Design review of the part built by this model. Coordinates are the model's own, in mm. Face numbers are marked on the shaded views. A direction names the side the tool comes from. Give positions to 0.01 mm unless a question says otherwise; leave off trailing zeros. Order: outer loops, then holes, each group sorted by start corner. A loop starts at its lowest first (then second) coordinate and runs counter-clockwise, first axis right, second up. Notation, with made-up numbers: (61.5, 36.5) -> (104.5, 36.5) arc R11 cw to (104.5, 53.5) -> close; hole circle Ø8 at (18, 71.5). An arc over 180 degrees is marked (long way). One line per item, written item: value.
from build123d import *

# Parameters (mm, degrees)
EXTRUDE_1_DEPTH     = 90
CUT_EXTRUDE_START   = -65
CUT_EXTRUDE_2_DEPTH = 65
SKETCH_4_R          = 2.1
CUT_EXTRUDE_3_DEPTH = 10


with BuildPart() as part:
    # Эскиз1 → Вытянуть1 (new body)
    with BuildSketch(Plane.XY):
        with BuildLine():
            Line((-17.5, 6.5), (-14.5, 6.5))
            ThreePointArc((-14.5, 6.5), (-13.792893219, 6.207106781), (-13.5, 5.5))
            Line((-13.5, 5.5), (-13.5, 2))
            ThreePointArc((-13.5, 2), (-12.914213562, 0.585786438), (-11.5, 0))
            Line((-11.5, 0), (11.5, 0))
            ThreePointArc((11.5, 0), (12.914213562, 0.585786438), (13.5, 2))
            Line((13.5, 2), (13.5, 5.5))
            ThreePointArc((13.5, 5.5), (13.792893219, 6.207106781), (14.5, 6.5))
            Line((14.5, 6.5), (17.5, 6.5))
            Line((17.5, 6.5), (17.5, 7.5))
            Line((17.5, 7.5), (14.5, 7.5))
            ThreePointArc((14.5, 7.5), (13.085786438, 6.914213562), (12.5, 5.5))
            Line((12.5, 5.5), (12.5, 2))
            ThreePointArc((12.5, 2), (12.207106781, 1.292893219), (11.5, 1))
            Line((11.5, 1), (-11.5, 1))
            ThreePointArc((-11.5, 1), (-12.207106781, 1.292893219), (-12.5, 2))
            Line((-12.5, 2), (-12.5, 5.5))
            ThreePointArc((-12.5, 5.5), (-13.085786438, 6.914213562), (-14.5, 7.5))
            Line((-14.5, 7.5), (-17.5, 7.5))
            Line((-17.5, 7.5), (-17.5, 6.5))
        make_face()
    extrude(amount=EXTRUDE_1_DEPTH)

    # Эскиз3 → Вырез-Вытянуть2 (cut)
    with BuildSketch(Plane.XY.offset(90).offset(CUT_EXTRUDE_START)):
        with BuildLine():
            Line((-17.5, 7.5), (-17.5, 6.5))
            Line((-17.5, 6.5), (-14.5, 6.5))
            ThreePointArc((-14.5, 6.5), (-13.792893219, 6.207106781), (-13.5, 5.5))
            Line((-13.5, 5.5), (-13.5, 2))
            ThreePointArc((-13.5, 2), (-12.914213562, 0.585786438), (-11.5, 0))
            Line((-11.5, 0), (11.5, 0))
            ThreePointArc((11.5, 0), (12.914213562, 0.585786438), (13.5, 2))
            Line((13.5, 2), (13.5, 5.5))
            ThreePointArc((13.5, 5.5), (13.792893219, 6.207106781), (14.5, 6.5))
            Line((14.5, 6.5), (17.5, 6.5))
            Line((17.5, 6.5), (17.5, 7.5))
            Line((17.5, 7.5), (14.5, 7.5))
            ThreePointArc((14.5, 7.5), (13.085786438, 6.914213562), (12.5, 5.5))
            Line((12.5, 5.5), (12.5, 2))
            ThreePointArc((12.5, 2), (12.207106781, 1.292893219), (11.5, 1))
            Line((11.5, 1), (-11.5, 1))
            ThreePointArc((-11.5, 1), (-12.207106781, 1.292893219), (-12.5, 2))
            Line((-12.5, 2), (-12.5, 5.5))
            ThreePointArc((-12.5, 5.5), (-13.085786438, 6.914213562), (-14.5, 7.5))
            Line((-14.5, 7.5), (-17.5, 7.5))
        make_face()
    extrude(amount=CUT_EXTRUDE_2_DEPTH, mode=Mode.SUBTRACT)

    # Эскиз4 → Вырез-Вытянуть3 (cut)
    with BuildSketch(Plane(origin=(0, 1, 0), x_dir=(-1, 0, 0), z_dir=(0, 1, 0))):
        with Locations((7.5, 7.5)):
            Circle(SKETCH_4_R)
        with Locations((-7.5, 17.5)):
            Circle(SKETCH_4_R)
    extrude(amount=-CUT_EXTRUDE_3_DEPTH, mode=Mode.SUBTRACT)


solid = part.part
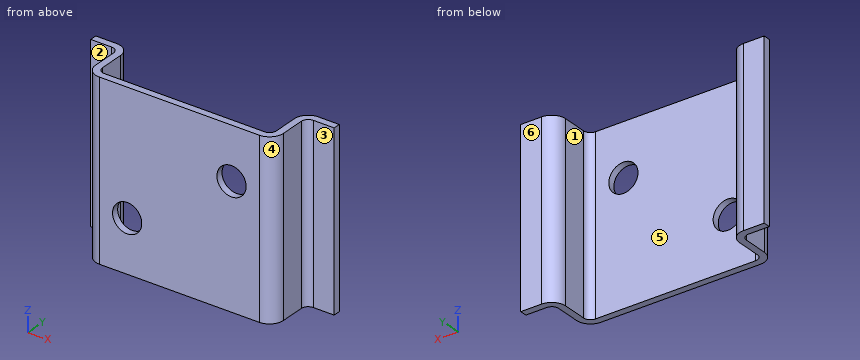
Item 1: Add section D-D on z = 4. Give the boundary of the cut face in (x, y).
Returned:
outline: (-17.5, 6.5) -> (-14.5, 6.5) arc R1 cw to (-13.5, 5.5) -> (-13.5, 2) arc R2 ccw to (-11.5, 0) -> (11.5, 0) arc R2 ccw to (13.5, 2) -> (13.5, 5.5) arc R1 cw to (14.5, 6.5) -> (17.5, 6.5) -> (17.5, 7.5) -> (14.5, 7.5) arc R2 ccw to (12.5, 5.5) -> (12.5, 2) arc R1 cw to (11.5, 1) -> (-11.5, 1) arc R1 cw to (-12.5, 2) -> (-12.5, 5.5) arc R2 ccw to (-14.5, 7.5) -> (-17.5, 7.5) -> close
Item 2: Draft analysis for pull direction X (two halves, no side actions). For the marked faces 4, 5 and 6, state which applies: pulls with the +X half, pulls with the -X half, needs draft (parallel to the pull), parting line crosses it, or undercut.
Returned:
face 4: pulls with the +X half
face 5: undercut
face 6: needs draft
Item 3: Add section C-C on x = -7.5. Give the boundary of the cut face in (y, z), plus the area to 3 significant figures.
Returned:
outline: (0, 0) -> (1, 0) -> (1, 5.4) -> (0, 5.4) -> close; (0, 9.6) -> (1, 9.6) -> (1, 25) -> (0, 25) -> close
area: 20.8 mm²
Item 4: Clearance check with flat-ended pins moving along their axes: P1, Ø3, axis at y = 4.5, z = 7, coming from the -X side; P2, Ø1, axis at x = -4, z = 16, coming from the +Y side; P3, Ø3.5, axis at x = -16.5, z = 14, coming from the -Y side. State where each tip first meets the part, or that it passes through.
Returned:
P1: x = -13.63
P2: y = 1
P3: y = 6.5
Item 5: Add section B-B on z = 7.5. Give the boundary of the cut face in (x, y), plus the area to 3 significant figures.
Returned:
outline: (-17.5, 6.5) -> (-14.5, 6.5) arc R1 cw to (-13.5, 5.5) -> (-13.5, 2) arc R2 ccw to (-11.5, 0) -> (-9.6, 0) -> (-9.6, 1) -> (-11.5, 1) arc R1 cw to (-12.5, 2) -> (-12.5, 5.5) arc R2 ccw to (-14.5, 7.5) -> (-17.5, 7.5) -> close; (-5.4, 0) -> (11.5, 0) arc R2 ccw to (13.5, 2) -> (13.5, 5.5) arc R1 cw to (14.5, 6.5) -> (17.5, 6.5) -> (17.5, 7.5) -> (14.5, 7.5) arc R2 ccw to (12.5, 5.5) -> (12.5, 2) arc R1 cw to (11.5, 1) -> (-5.4, 1) -> close
area: 41.2 mm²
Item 6: Add section A-A on y = 4.75. Give the boundary of the cut face in (x, z), plus the area to 3 significant figures.
Returned:
outline: (-13.5, 0) -> (-12.5, 0) -> (-12.5, 25) -> (-13.5, 25) -> close; (12.5, 0) -> (13.5, 0) -> (13.5, 25) -> (12.5, 25) -> close
area: 50.0 mm²
Item 7: Machinability: for the marked faces 1, 2 and 3, which of the approach directions +Z, -Z, +X, -X, +Y, -Y give a long, thin tool a straight path to every point of the face, cutting with its end or side? Answer none if there is none.
Returned:
face 1: +Z, -Z, +Y
face 2: +Z, -Z, -X, -Y
face 3: +Z, -Z, +X, -Y
Item 8: To check wall thickness, follow line 1 along X through (y, z) = (4, 5); line 2 along Z through (x, y) = (-7.5, 0.7); line 3 along Z through (x, y) = (7.5, 0.45). State the ranges of each line that lie inside material, in increasing order. Write a range as from..to.
Returned:
line 1: -13.5..-12.5, 12.5..13.5
line 2: 0..5.4, 9.6..25
line 3: 0..15.4, 19.6..25
